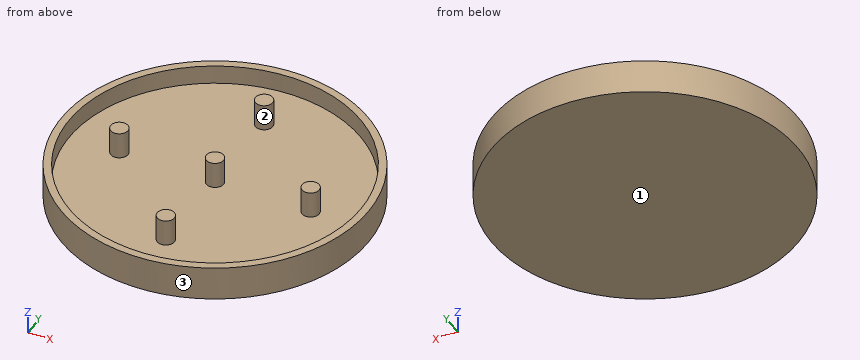
```python
from build123d import *

# Parameters (mm, degrees)
F0_R     = 40
F0_R_2   = 38
F1_DEPTH = 9
F2_DEPTH = 4
F3_R     = 2.25
F4_DEPTH = 7


with BuildPart() as f1:
    # F0 (on Top) → F1 (new body)
    with BuildSketch(Plane.XY):
        Circle(F0_R)
        Circle(F0_R_2, mode=Mode.SUBTRACT)
    extrude(amount=F1_DEPTH)

    # F0 (on Top) → F2 (join)
    with BuildSketch(Plane.XY):
        Circle(F0_R_2)
    extrude(amount=F2_DEPTH)

    # F3 (on face) → F4 (join)
    with BuildSketch(Plane.XY.offset(4)):
        Circle(F3_R)
        with Locations((-25, 0)):
            Circle(F3_R)
        with Locations((25, 0)):
            Circle(F3_R)
        with Locations((0, 25)):
            Circle(F3_R)
        with Locations((0, -25)):
            Circle(F3_R)
    extrude(amount=F4_DEPTH)


solid = f1.part
```
Input: part model. Units: mm. Frame: model coordinates. Face numbers are marked on the shaded views. Coordinates: 2 decimals unless noted, no trailing zeros. Loops run counter-clockwise (first coordinate to the right, second up) from the corner with the lowest first, then second, coordinate; pieces in that order, holes last.
Q1. Section A-A, the plane z = 5.5. Return the cut outline in (x, y).
Results are:
outline: circle Ø80 at (0, 0); circle Ø4.5 at (-25, 0); circle Ø4.5 at (0, -25); circle Ø4.5 at (0, 0); circle Ø4.5 at (0, 25); circle Ø4.5 at (25, 0); hole circle Ø76 at (0, 0)
Q2. Line query: line 1 along Y through (x, z) = (0, 5.4); line 2 along X through (y, z) = (-26.5, 7); line 3 along Z through (x, y) = (2, 34). Output: solid intervals per line, ascending.
Results are:
line 1: y = -40 to -38, -27.25 to -22.75, -2.25 to 2.25, 22.75 to 27.25, 38 to 40
line 2: x = -29.96 to -27.24, -1.68 to 1.68, 27.24 to 29.96
line 3: z = 0 to 4
Q3. Mould query, pull axis Y, two halves, no side actions, for the marked faces 1, 2 and 3. Classes: +Y half, -Y half, draft (parallel to the pull), parting line (faces both ways), or undercut.
Results are:
face 1: draft
face 2: undercut
face 3: parting line
Q4. Contact query for flat-ended pins moving along their axis: pin 1 (1 mm diameter, centred on x = 23, z = 7, fed in from -Y); pin 2 (6 mm diameter, centred on y = -7, z = 5, fed in from -X); pin 3 (3 mm diameter, centred on x = 11.5, y = -20, fed in from +Z). Output: stop coordinate, or through.
Results are:
pin 1: stops at y = -33.07
pin 2: stops at x = -39.8
pin 3: stops at z = 4
Q5. Section D-D, the plane z = 10. Return the cut outline in (x, y), and give its area (3 significant figures).
Results are:
outline: circle Ø4.5 at (-25, 0); circle Ø4.5 at (0, -25); circle Ø4.5 at (0, 0); circle Ø4.5 at (0, 25); circle Ø4.5 at (25, 0)
area: 79.5 mm2
Q6. Section B-B, the plane x = 0. Return the cut outline in (y, z), and give its area (4 significant figures).
Results are:
outline: (-40, 0) - (40, 0) - (40, 9) - (38, 9) - (38, 4) - (27.25, 4) - (27.25, 11) - (22.75, 11) - (22.75, 4) - (2.25, 4) - (2.25, 11) - (-2.25, 11) - (-2.25, 4) - (-22.75, 4) - (-22.75, 11) - (-27.25, 11) - (-27.25, 4) - (-38, 4) - (-38, 9) - (-40, 9) - close
area: 434.5 mm2
